from build123d import *

# Parameters (mm, degrees)
SKETCH_1_W          = 38
SKETCH_1_H          = 300
EXTRUDE_1_DEPTH     = 1.2
CUT_EXTRUDE_1_DEPTH = 1.2


with BuildPart() as part:
    # Эскиз1 → Бобышка-Вытянуть1 (new body)
    with BuildSketch(Plane.XY):
        Rectangle(SKETCH_1_W, SKETCH_1_H)
    extrude(amount=EXTRUDE_1_DEPTH)

    # Эскиз2 → Вырез-Вытянуть1 (cut)
    with BuildSketch(Plane.XY.offset(1.2)):
        with BuildLine():
            ThreePointArc((0, -114.945517328), (-3.6, -118.545517328), (0, -122.145517328))
            Line((0, -122.145517328), (0, -114.945517328))
        make_face()
        with BuildLine():
            Line((0, -114.945517328), (0, -122.145517328))
            ThreePointArc((0, -122.145517328), (2.545584412, -121.09110174), (3.6, -118.545517328))
            ThreePointArc((3.6, -118.545517328), (2.545584412, -115.999932916), (0, -114.945517328))
        make_face()
        with BuildLine():
            ThreePointArc((-5.9, -135), (-9.5, -131.4), (-13.1, -135))
            Line((-13.1, -135), (-5.9, -135))
        make_face()
        with BuildLine():
            Line((-5.9, -135), (-13.1, -135))
            ThreePointArc((-13.1, -135), (-9.5, -138.6), (-5.9, -135))
        make_face()
        with BuildLine():
            ThreePointArc((13.1, -135), (9.5, -131.4), (5.9, -135))
            Line((5.9, -135), (13.1, -135))
        make_face()
        with BuildLine():
            Line((13.1, -135), (5.9, -135))
            ThreePointArc((5.9, -135), (9.5, -138.6), (13.1, -135))
        make_face()
    extrude(amount=-CUT_EXTRUDE_1_DEPTH, mode=Mode.SUBTRACT)


solid = part.part
The model under review builds one solid part; all positions refer to its coordinate system, in mm. Coordinates: 2 decimals unless noted, no trailing zeros. Order: outer loops, then holes, each group sorted by start corner. A loop starts at its lowest first (then second) coordinate and runs counter-clockwise, first axis right, second up. Notation, with made-up numbers: (31, 65.5) -> (72, 65.5) arc R13 cw to (72, 73.5) -> close; hole circle Ø9 at (19, 64). An arc over 180 degrees is marked (long way). Answer in a Markdown table with one row per item.
(1) Insertion check: pin 1 (6 mm diameter, centred on x = -9.5, y = -135, fed in from +Z). The pin has a flat end and moves straight along its axis. Give the tip position at first contact, or say it passes through.
Answers:
| item | result |
|---|---|
| pin 1 | through |
(2) The part is to be moulded in two halves that separate along Y. For faces 1 (the flat face through (0, 2, 0)), 2 (the cylindrical face through (6.175, -133.621, 0.608)), say which applies: +Y half, -Y half, draft (parallel to the pull), parting line (faces both ways), or undercut.
Answers:
| item | result |
|---|---|
| face 1 | draft |
| face 2 | undercut |
(3) Consider section A-A (x = -9.5). Write out the cut boundary in (y, z).
Answers:
| item | result |
|---|---|
| outline | (-150, 0) -> (-138.6, 0) -> (-138.6, 1.2) -> (-150, 1.2) -> close; (-131.4, 0) -> (150, 0) -> (150, 1.2) -> (-131.4, 1.2) -> close |
(4) Consider section B-B (y = -135). Write out the cut boundary in (x, z).
Answers:
| item | result |
|---|---|
| outline | (-19, 0) -> (-13.1, 0) -> (-13.1, 1.2) -> (-19, 1.2) -> close; (-5.9, 0) -> (5.9, 0) -> (5.9, 1.2) -> (-5.9, 1.2) -> close; (13.1, 0) -> (19, 0) -> (19, 1.2) -> (13.1, 1.2) -> close |
(5) Wall thickness on line 1 along X through (y, z) = (-135, 0.2); line 2 along Y through (x, z) = (9.5, 0.6); line 3 along Y through (x, z) = (-11, 0.85): over which ranges is each line inside the solid? List them lowest first.
Answers:
| item | result |
|---|---|
| line 1 | -19 to -13.1, -5.9 to 5.9, 13.1 to 19 |
| line 2 | -150 to -138.6, -131.4 to 150 |
| line 3 | -150 to -138.27, -131.73 to 150 |
